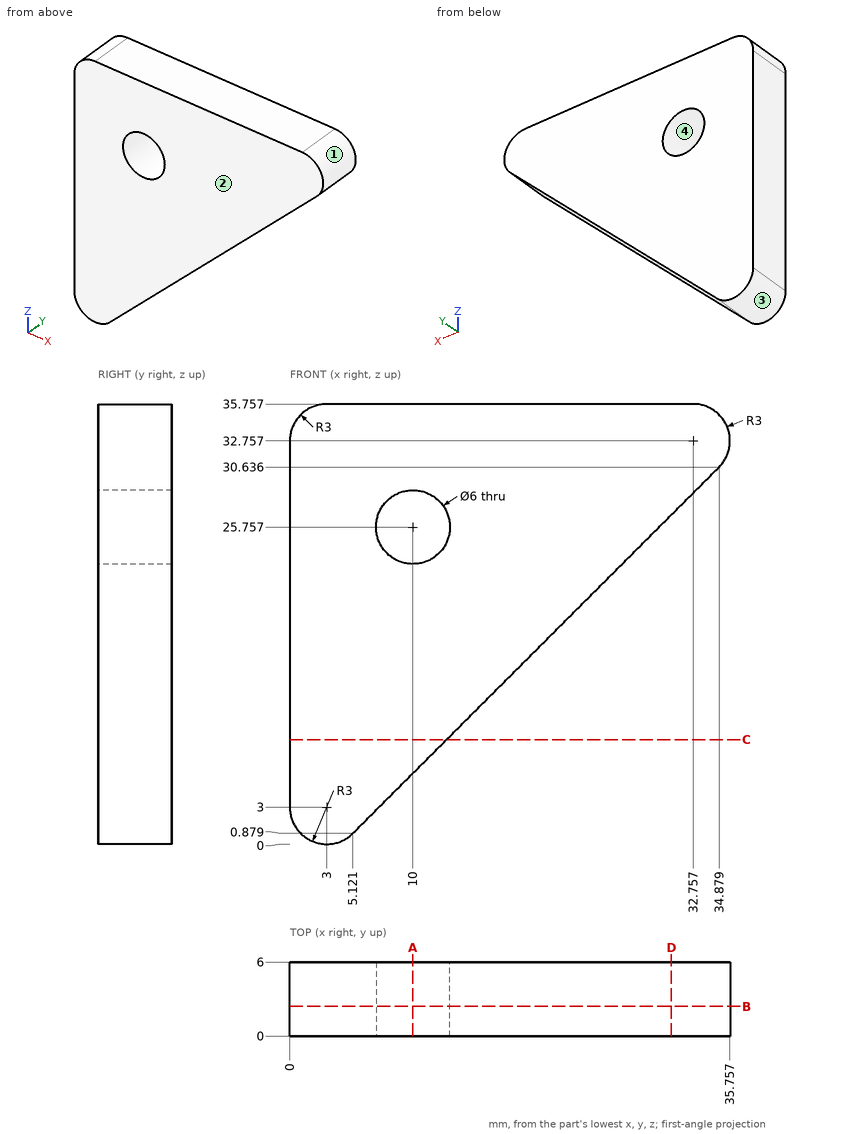
Here's the drawing with two shaded views (mm, measured from the low corner). I have some questions. Round coordinates to 2 decimals unless told otherwise and drop trailing zeros. Order: outer loops, then holes, each group sorted by start corner. A loop starts at its lowest first (then second) coordinate and runs counter-clockwise, first axis right, second up. Notation, with made-up numbers: (10.25, 45) -> (15.25, 45) arc R13 ccw to (15.25, 62) -> close; hole circle Ø6 at (51.5, 72.5). An arc over 180 degrees is marked (long way). Write each question's results on one line, items separated by ' | '. Start each with the question number.
Item 1: If we section it at A-A, the plane x = 10: Write out the boundary of the cut face in (y, z), then the cut area to 3 significant figures.
Item 2: Thinking about a two-plate mould opening in Z: for the marked faces 1, 2, 3 and 4, which applies, +Z half, -Z half, draft (parallel to the pull), parting line (faces both ways), or undercut?
Item 3: If we section it at D-D, the plane x = 31: Write out the boundary of the cut face in (y, z), then the cut area to 3 significant figures.
Item 4: Please list where these lines run through material, in increasing order: L1, parallel to X at y = 3.95, z = 27; L2, parallel to Z at x = 10, y = 3.55; L3, parallel to X at y = 4.95, z = 24.5 (1 decimal).
Item 5: If we section it at C-C, the plane z = 8.5: Write out the boundary of the cut face in (x, y).
Item 6: If we section it at B-B, the plane y = 2.4: Write out the boundary of the cut face in (x, z).
Results:
1) outline: (0, 5.76) -> (6, 5.76) -> (6, 22.76) -> (0, 22.76) -> close; (0, 28.76) -> (6, 28.76) -> (6, 35.76) -> (0, 35.76) -> close | area: 144 mm2
2) face 1: parting line | face 2: draft | face 3: -Z half | face 4: undercut
3) outline: (0, 26.76) -> (6, 26.76) -> (6, 35.76) -> (0, 35.76) -> close | area: 54.0 mm2
4) L1: x = 0 to 7.27, 12.73 to 31.24 | L2: z = 5.76 to 22.76, 28.76 to 35.76 | L3: x = 0 to 7.3, 12.7 to 28.7
5) outline: (0, 0) -> (12.74, 0) -> (12.74, 6) -> (0, 6) -> close
6) outline: (0, 3) arc R3 ccw to (5.12, 0.88) -> (34.88, 30.64) arc R3 ccw to (32.76, 35.76) -> (3, 35.76) arc R3 ccw to (0, 32.76) -> close; hole circle Ø6 at (10, 25.76)
